Design review of the part built by this model. Coordinates are the model's own, in mm. A direction names the side the tool comes from. Coordinates: 2 decimals unless noted, no trailing zeros. Order: outer loops, then holes, each group sorted by start corner. A loop starts at its lowest first (then second) coordinate and runs counter-clockwise, first axis right, second up. Notation, with made-up numbers: (-5, 39) -> (8, 39) arc R23 ccw to (8, 63) -> close; hole circle Ø3 at (-22, 89.25). An arc over 180 degrees is marked (long way). Use a Markdown table: item, result. Add a question column.
Q1. The part is to be moulded in two halves that separate along Y. For faces 4 (the face through (-3.479, 16.744, 16.369)), 5 (the face through (-3.479, -16.869, 16.244)), 6 (the face through (-6, 16.15, -1)), say which applies: pulls with the +Y half, pulls with the -Y half, needs draft (parallel to the pull), parting line crosses it, or undercut.
Q2. Insertion check: pin 1 (9.5 mm diameter, centred on y = 4.5, z = 5, fed in from -X); pin 2 (2 mm diameter, centred on x = -2.5, z = -13.5, fed in from +Y); pin 3 (2.5 mm diameter, centred on x = -6, z = 3, fed in from +Y). Each pin has a flat end and moves straight along its axis. Give the tip position at first contact, or say it passes through.
Q3. Add section A-A (z = -0.5). State the section outline as (x, y) points, then the cut area to 3 significant figures.
Q4. Add section C-C (x = -6.25). State the section outline as (y, z) points.
Q5. Machinability: for faces 1 (the face through (-3.479, 16.869, -17.244)), 2 (the face through (-6.46, 14.72, 14.15)), 3 (the face through (-1.01, -0.27, -19.19)), which of the approach directions +Z, -Z, +X, -X, +Y, -Y give a long, thin tool a straight path to every point of the face, cutting with its end or side? Answer none if there is none.
Q6. Add section B-B (y = 21.5). State the section outline as (x, z) points, then the cut area to 3 significant figures.
Q7. Wall thickness on probe 1 along X at (y, z) = (14.5, 2.5); probe 2 along Y at (x, z) = (-4.5, -9); probe 3 along Z at (x, y) = (-5, 6.5): over which ranges is each line inside the solid? List them lowest first.
Q8. Add section D-D (y = -2). State the section outline as (x, z) points.
from build123d import *

# Parameters (mm, degrees)
F1_DEPTH = 2
F2_DEPTH = 4
F4_W     = 23.5562745947
F4_H     = 63.5293796659
F5_DEPTH = 3.5651598846
F7_DEPTH = 5
F8_SIZE2 = 0.5
F8_SIZE  = 4
F9_D     = 2.2


with BuildPart() as f1:
    # F0 (on Right) → F1 (new body)
    with BuildSketch(Plane.YZ):
        with BuildLine():
            Line((11.15, 21.65), (-11.15, 21.65))
            ThreePointArc((-11.15, 21.65), (-18.9281745931, 18.4281745931), (-22.15, 10.65))
            Line((-22.15, 10.65), (-22.15, -11.65))
            ThreePointArc((-22.15, -11.65), (-18.9281745931, -19.4281745931), (-11.15, -22.65))
            Line((-11.15, -22.65), (11.15, -22.65))
            ThreePointArc((11.15, -22.65), (18.9281745931, -19.4281745931), (22.15, -11.65))
            Line((22.15, -11.65), (22.15, 10.65))
            ThreePointArc((22.15, 10.65), (18.9281745931, 18.4281745931), (11.15, 21.65))
        make_face()
        with BuildLine():
            ThreePointArc((-19.15, 10.65), (-16.8068542495, 16.3068542495), (-11.15, 18.65))
            Line((-11.15, 18.65), (11.15, 18.65))
            ThreePointArc((11.15, 18.65), (16.8068542495, 16.3068542495), (19.15, 10.65))
            Line((19.15, 10.65), (19.15, -11.65))
            ThreePointArc((19.15, -11.65), (16.8068542495, -17.3068542495), (11.15, -19.65))
            Line((11.15, -19.65), (-11.15, -19.65))
            ThreePointArc((-11.15, -19.65), (-16.8068542495, -17.3068542495), (-19.15, -11.65))
            Line((-19.15, -11.65), (-19.15, 10.65))
        make_face(mode=Mode.SUBTRACT)
        with BuildLine():
            Line((11.15, 18.65), (-11.15, 18.65))
            ThreePointArc((-11.15, 18.65), (-16.8068542495, 16.3068542495), (-19.15, 10.65))
            Line((-19.15, 10.65), (-19.15, -11.65))
            ThreePointArc((-19.15, -11.65), (-16.8068542495, -17.3068542495), (-11.15, -19.65))
            Line((-11.15, -19.65), (11.15, -19.65))
            ThreePointArc((11.15, -19.65), (16.8068542495, -17.3068542495), (19.15, -11.65))
            Line((19.15, -11.65), (19.15, 10.65))
            ThreePointArc((19.15, 10.65), (16.8068542495, 16.3068542495), (11.15, 18.65))
        make_face()
        Polygon((-22.15, -11.65), (-22.15, 10.65), (-24.15, 8.65), (-24.15, -9.65), align=None)
        Polygon((24.15, 8.65), (22.15, 10.65), (22.15, -11.65), (24.15, -9.65), align=None)
    extrude(amount=-F1_DEPTH)

    # F0 (on Right) → F2 (join)
    with BuildSketch(Plane.YZ):
        with BuildLine():
            Line((11.15, 18.65), (-11.15, 18.65))
            ThreePointArc((-11.15, 18.65), (-16.8068542495, 16.3068542495), (-19.15, 10.65))
            Line((-19.15, 10.65), (-19.15, -11.65))
            ThreePointArc((-19.15, -11.65), (-16.8068542495, -17.3068542495), (-11.15, -19.65))
            Line((-11.15, -19.65), (11.15, -19.65))
            ThreePointArc((11.15, -19.65), (16.8068542495, -17.3068542495), (19.15, -11.65))
            Line((19.15, -11.65), (19.15, 10.65))
            ThreePointArc((19.15, 10.65), (16.8068542495, 16.3068542495), (11.15, 18.65))
        make_face()
    extrude(amount=-F2_DEPTH)

    # F4 (on face) → F5 (cut, through all)
    with BuildSketch(Plane(origin=(7.1691742633, 0, -15.3743438221), x_dir=(0.906307787, 0, 0.4226182617), z_dir=(0.4226182617, 0, -0.906307787))):
        with Locations((-8.6737343809, -4.5895911753)):
            Rectangle(F4_W, F4_H)
    extrude(amount=F5_DEPTH, mode=Mode.SUBTRACT)

    # F6 (on face) → F7 (join)
    with BuildSketch(Plane(origin=(-4, 0, 0), x_dir=(0, -1, 0), z_dir=(-1, 0, 0))):
        with BuildLine():
            ThreePointArc((19.15, 10.65), (16.8068542495, 16.3068542495), (11.15, 18.65))
            Line((11.15, 18.65), (-11.15, 18.65))
            ThreePointArc((-11.15, 18.65), (-16.8068542495, 16.3068542495), (-19.15, 10.65))
            Line((-19.15, 10.65), (-19.15, -11.65))
            ThreePointArc((-19.15, -11.65), (-16.8068542495, -17.3068542495), (-11.15, -19.65))
            Line((-11.15, -19.65), (11.15, -19.65))
            ThreePointArc((11.15, -19.65), (16.8068542495, -17.3068542495), (19.15, -11.65))
            Line((19.15, -11.65), (19.15, 10.65))
        make_face()
        with BuildLine():
            ThreePointArc((11.15, 15.65), (14.6855339059, 14.1855339059), (16.15, 10.65))
            Line((16.15, 10.65), (16.15, -11.65))
            ThreePointArc((16.15, -11.65), (14.6855339059, -15.1855339059), (11.15, -16.65))
            Line((11.15, -16.65), (-11.15, -16.65))
            ThreePointArc((-11.15, -16.65), (-14.6855339059, -15.1855339059), (-16.15, -11.65))
            Line((-16.15, -11.65), (-16.15, 10.65))
            ThreePointArc((-16.15, 10.65), (-14.6855339059, 14.1855339059), (-11.15, 15.65))
            Line((-11.15, 15.65), (11.15, 15.65))
        make_face(mode=Mode.SUBTRACT)
    extrude(amount=F7_DEPTH)

    # F8
    f8_edges = [f1.edges().sort_by_distance(p)[0] for p in [
        (-9, -16.806854, -17.306854),
        (-9, 0, -19.65),
        (-9, -19.15, -0.5),
    ]]
    chamfer(f8_edges, length=F8_SIZE, length2=F8_SIZE2)

    # F9 (through all)
    with Locations(Plane.YZ):
        with Locations((-21.4, -0.5), (21.4, -0.5)):
            Hole(F9_D / 2)


solid = f1.part
Established:
| question | item | result |
|---|---|---|
| 1 | face 4 | pulls with the +Y half |
| 1 | face 5 | pulls with the -Y half |
| 1 | face 6 | undercut |
| 2 | pin 1 | x = -4 |
| 2 | pin 2 | y = 22.11 |
| 2 | pin 3 | y = 19.15 |
| 3 | outline | (-9, -18.65) -> (-5, -19.15) -> (-2, -19.15) -> (-2, -20.3) -> (0, -20.3) -> (0, 20.3) -> (-2, 20.3) -> (-2, 19.15) -> (-5, 19.15) -> (-9, 18.65) -> (-9, 16.15) -> (-4, 16.15) -> (-4, -16.15) -> (-9, -16.15) -> close; (-2, -24.15) -> (0, -24.15) -> (0, -22.5) -> (-2, -22.5) -> close; (-2, 22.5) -> (0, 22.5) -> (0, 24.15) -> (-2, 24.15) -> close |
| 3 | area | 192 mm^2 |
| 4 | outline | (-18.99, -11.65) arc R7.84 ccw to (-11.15, -19.49) -> (11.15, -19.49) arc R7.84 ccw to (18.99, -11.65) -> (18.99, 10.65) arc R7.84 ccw to (11.15, 18.49) -> (-11.15, 18.49) arc R7.84 ccw to (-18.99, 10.65) -> close; hole (-16.15, -11.65) arc R5 ccw to (-11.15, -16.65) -> (11.15, -16.65) arc R5 ccw to (16.15, -11.65) -> (16.15, 10.65) arc R5 ccw to (11.15, 15.65) -> (-11.15, 15.65) arc R5 ccw to (-16.15, 10.65) -> close |
| 5 | face 1 | -Z, -X, +Y |
| 5 | face 2 | -X |
| 5 | face 3 | -Z, +X, +Y, -Y |
| 6 | outline | (-2, -15.38) -> (0, -15.38) -> (0, -1.6) -> (-2, -1.6) -> close; (-2, 0.6) -> (0, 0.6) -> (0, 14.38) -> (-2, 14.38) -> close |
| 6 | area | 55.1 mm^2 |
| 7 | probe 1 | -4 to 0 |
| 7 | probe 2 | -19.15 to -16.15, 16.15 to 19.15 |
| 7 | probe 3 | -19.65 to -16.65, 15.65 to 18.65 |
| 8 | outline | (-9, -19.15) -> (-5, -19.65) -> (-2, -19.65) -> (0, -18.72) -> (0, 21.65) -> (-2, 21.65) -> (-2, 18.65) -> (-5, 18.65) -> (-9, 18.15) -> (-9, 15.65) -> (-4, 15.65) -> (-4, -16.65) -> (-9, -16.65) -> close |
